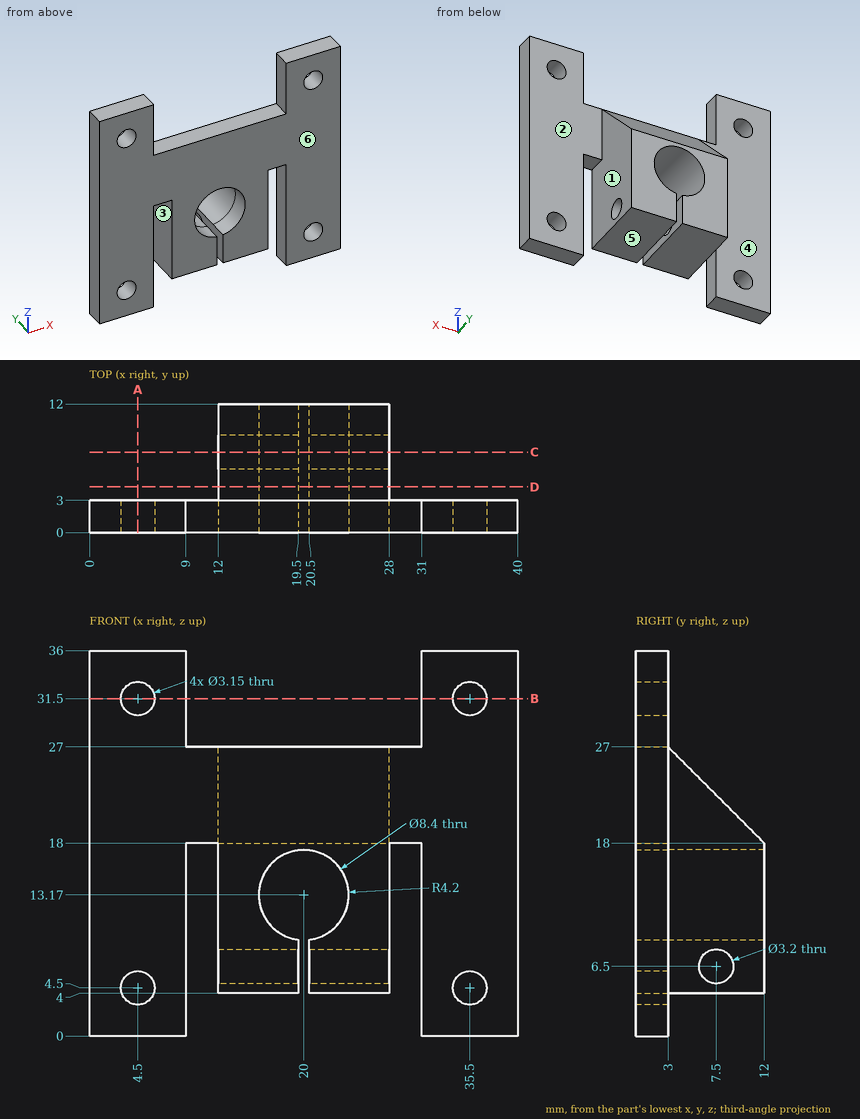
Print and shaded views of the part. All mm, measured from the part's lowest x, y and z. A direction names the side the tool comes from. Coordinates: 2 decimals unless noted, no trailing zeros. Order: outer loops, then holes, each group sorted by start corner. A loop starts at its lowest first (then second) coordinate and runs counter-clockwise, first axis right, second up. Notation, with made-up numbers: M 85,-0.5 L 142,-0.5 A26 cw 142,20.5 Z; hole C 21.5,2 d3. An arc over 180 degrees is marked long. One line per question, with ' | ' between items. Start each with the question number.
Q1. Probe L1, parallel to X at y = 1.1, z = 4.5 (3 decimals); L2, parallel to X at y = 1.5, z = 17.5; L3, parallel to X at y = 1.1, z = 31.5 (3 decimals). List the from-to ranges inside material, lowest first. Write a range as from..to.
Q2. Two-plate mould, pull along X, no slides. Class the marked faces 1, 2 and 3: +X half, -X half, draft (parallel to the pull), parting line (faces both ways), or undercut.
Q3. Saw through at C-C (y = 7.5). List the corners of the cut face in (x, z).
Q4. Saw through at A-A (x = 4.5). List the corners of the cut face in (y, z) (3 decimals), then the cut area to 3 significant figures.
Q5. Saw through at B-B (z = 31.5). List the corners of the cut face in (x, y) (3 decimals), then the cut area to 3 significant figures.
Q6. Saw through at D-D (y = 4.25). List the corners of the cut face in (x, z).
Q7. 3-axis set-ups, long thin cutter, end or side, ignore diameter. For the marked faces 4, 5 and 6: which of +Z, -Z, +X, -X, +Y, -Y reach the whole face in a straight line?
Q8. Flat gauge pins, fed straight in: pin 1 Ø5 at (y, z) = (7, 10.5) entering from -X; pin 2 Ø5 at (x, y) = (22.5, 10) entering from +Z; pin 3 Ø10 at (x, z) = (31.5, 32.5) entering from +Y. Where does each tip first touch, or does it go through?
Check values:
1) L1: x = 0..2.925, 6.075..9, 12..19.5, 20.5..28, 31..33.925, 37.075..40 | L2: x = 0..9, 12..28, 31..40 | L3: x = 0..2.925, 6.075..9, 31..33.925, 37.075..40
2) face 1: undercut | face 2: draft | face 3: undercut
3) outline: M 12,4 L 19.5,4 L 19.5,4.9 L 12,4.9 Z; M 12,8.1 L 19.5,8.1 L 19.5,9 A4.2 cw long 20.5,9 L 20.5,8.1 L 28,8.1 L 28,22.5 L 12,22.5 Z; M 20.5,4 L 28,4 L 28,4.9 L 20.5,4.9 Z
4) outline: M 0,0 L 3,0 L 3,2.925 L 0,2.925 Z; M 0,6.075 L 3,6.075 L 3,29.925 L 0,29.925 Z; M 0,33.075 L 3,33.075 L 3,36 L 0,36 Z | area: 89.1 mm2
5) outline: M 0,0 L 2.925,0 L 2.925,3 L 0,3 Z; M 6.075,0 L 9,0 L 9,3 L 6.075,3 Z; M 31,0 L 33.925,0 L 33.925,3 L 31,3 Z; M 37.075,0 L 40,0 L 40,3 L 37.075,3 Z | area: 35.1 mm2
6) outline: M 12,4 L 19.5,4 L 19.5,9 A4.2 cw long 20.5,9 L 20.5,4 L 28,4 L 28,25.75 L 12,25.75 Z
7) face 4: +Z, -Z, -X, +Y | face 5: -Z, +Y, -Y | face 6: +Z, -Z, +X, -X, -Y
8) pin 1: stops at x = 12 | pin 2: stops at z = 22.5 | pin 3: stops at y = 3
